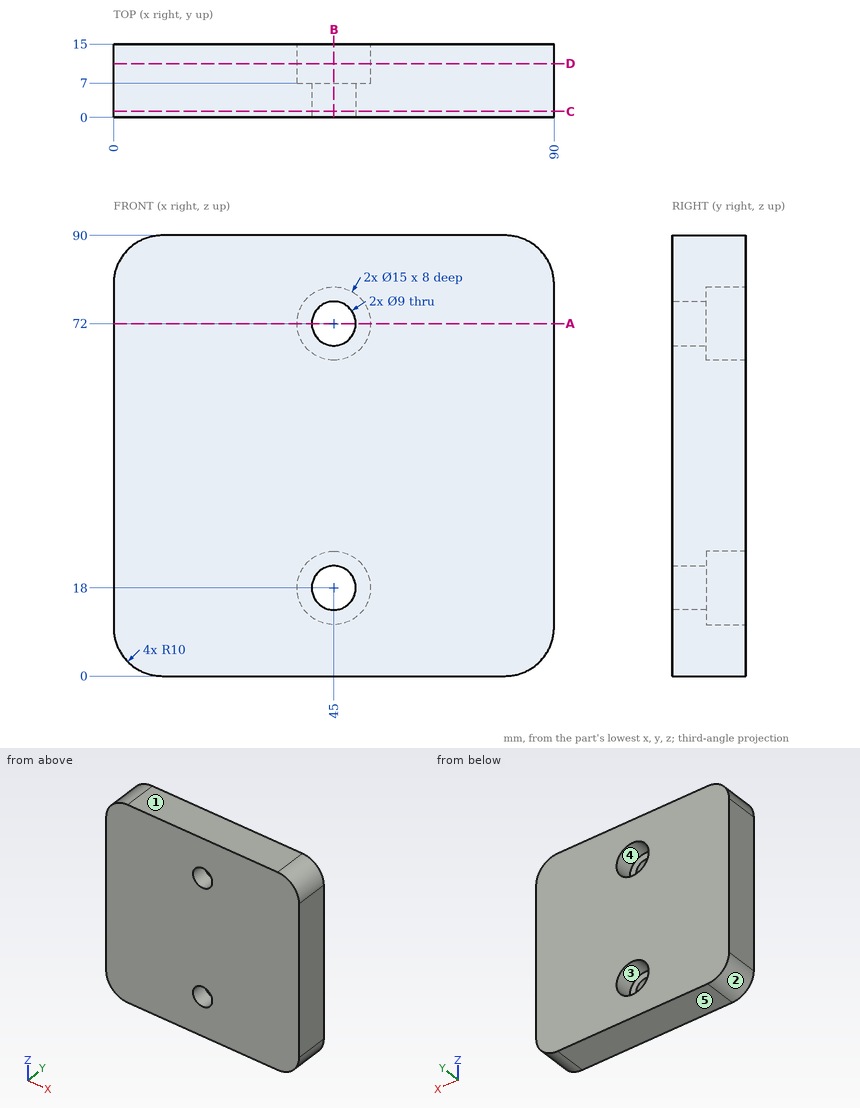
Part print with two shaded views. Sizes in mm from the minimum x, y, z corner. A direction names the side the tool comes from. Round coordinates to 2 decimals unless told otherwise and drop trailing zeros. Write each loop counter-clockwise with the first axis right and the second up, starting at its lowest first coordinate (ties: lowest second). Pieces come first, ordered by that corner, then holes. Notation, with made-up numbers: (-11.5, 35) -> (47.5, 35) arc R22 cw to (47.5, 44) -> close; hole circle Ø8 at (-28, -5.5). An arc over 180 degrees is marked (long way). Put each result on its own line as item: value.
Item 1: Wall check: probe 1 along X at (y, z) = (13.5, 72); probe 2 along Z at (x, y) = (44.5, 0.5); probe 3 along X at (y, z) = (1.5, 72). Give the ranges that are in metal, low to high. Write a range as from..to.
Here are the results:
probe 1: x = 0..37.5, 52.5..90
probe 2: z = 0..13.53, 22.47..67.53, 76.47..90
probe 3: x = 0..40.5, 49.5..90
Item 2: Tool access for the marked faces 4 and 5: list every direction of +Z, -Z, +X, -X, +Y, -Y with a clear straight run to the whole face (end or side of a thin tool).
Here are the results:
face 4: +Y
face 5: -Z, +X, -X, +Y, -Y
Item 3: Slice it at D-D, the plane y = 11. Give the cut face in (x, z), plus the area to 3 significant figures.
Here are the results:
outline: (0, 10) arc R10 ccw to (10, 0) -> (80, 0) arc R10 ccw to (90, 10) -> (90, 80) arc R10 ccw to (80, 90) -> (10, 90) arc R10 ccw to (0, 80) -> close; hole circle Ø15 at (45, 18); hole circle Ø15 at (45, 72)
area: 7,660 mm^2
Item 4: Flat gauge pin, fed straight in: P1, Ø4.5, axis at x = 48.5, z = 72, coming from the +Y side. Where does the tip first touch, or does it go through?
Here are the results:
P1: stops at y = 7
Item 5: Two-plate mould, pull along X, no slides. Class the marked faces 1, 2 and 3: pulls with the +X half, pulls with the -X half, needs draft (parallel to the pull), parting line crosses it, or undercut.
Here are the results:
face 1: needs draft
face 2: pulls with the -X half
face 3: undercut
Item 6: Slice it at A-A, the plane z = 72. Give the cut face in (x, y), plus the area to 3 significant figures.
Here are the results:
outline: (0, 0) -> (40.5, 0) -> (40.5, 7) -> (37.5, 7) -> (37.5, 15) -> (0, 15) -> close; (49.5, 0) -> (90, 0) -> (90, 15) -> (52.5, 15) -> (52.5, 7) -> (49.5, 7) -> close
area: 1,170 mm^2
Item 7: Slice it at C-C, the plane y = 1.25. Give the cut face in (x, z).
Here are the results:
outline: (0, 10) arc R10 ccw to (10, 0) -> (80, 0) arc R10 ccw to (90, 10) -> (90, 80) arc R10 ccw to (80, 90) -> (10, 90) arc R10 ccw to (0, 80) -> close; hole circle Ø9 at (45, 18); hole circle Ø9 at (45, 72)
Item 8: Slice it at B-B, the plane x = 45. Give the cut face in (y, z), plus the area to 3 significant figures.
Here are the results:
outline: (0, 0) -> (15, 0) -> (15, 10.5) -> (7, 10.5) -> (7, 13.5) -> (0, 13.5) -> close; (0, 22.5) -> (7, 22.5) -> (7, 25.5) -> (15, 25.5) -> (15, 64.5) -> (7, 64.5) -> (7, 67.5) -> (0, 67.5) -> close; (0, 76.5) -> (7, 76.5) -> (7, 79.5) -> (15, 79.5) -> (15, 90) -> (0, 90) -> close
area: 984 mm^2
